CAD build for the part. Positions are in the model's coordinates, mm. Face numbers are marked on the shaded views. A direction names the side the tool comes from. Give positions to 0.01 mm unless a question says otherwise; leave off trailing zeros. Loops run counter-clockwise (first coordinate to the right, second up) from the corner with the lowest first, then second, coordinate; pieces in that order, holes last.
Item 1: Saw through at A-A on z = 14.75. Give the cut face in (x, y) (3 decimals).
Item 2: Probe probe 1 along Z at (x, y) = (-235.5, -138.5); probe 2 along X at (y, z) = (15.5, 15); probe 3 along Z at (x, y) = (-219, -82.5). List the from-to ranges inside material, lowest first.
Item 3: Drop flat-ended pins along their axis: P1, Ø3, axis at x = -22.66, y = 14.67, coming from the +Z side; P2, Ø10, axis at x = -16.5, z = 10.5, coming from the +Y side; P3, Ø10, axis at y = -122.5, z = 9, coming from the +X side; P4, Ø1.9, axis at x = -22, y = 14, coming from the +Z side. Give the stop position or say it passes through.
Item 4: Which spindle directions (+Z, -Z, +X, -X, +Y, -Y) get a long thin tool onto all of the face, cutting with end or side? Do the marked faces 1, 2 and 3. Say none if no direction does.
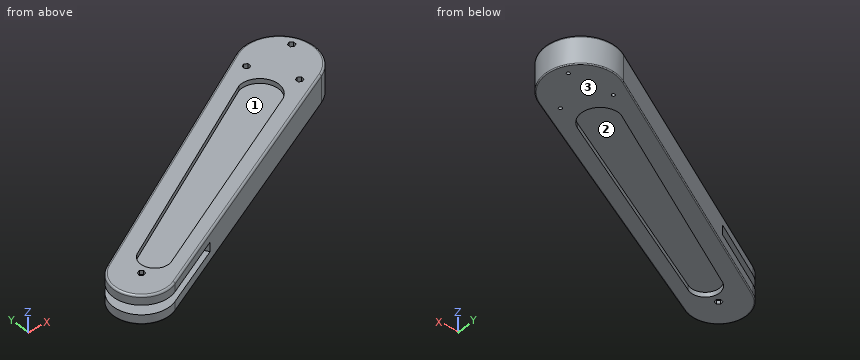
from build123d import *

# Parameters (mm, degrees)
BOSS_EXTRUDE1_DEPTH = 30
FILLET1_R           = 2
FILLET2_R           = 1
SKETCH6_W           = 100
SKETCH6_H           = 10
CUT_EXTRUDE3_DEPTH  = 129
CUT_EXTRUDE4_DEPTH  = 4
SKETCH8_R           = 1.9
CUT_EXTRUDE6_DEPTH  = 112
CUT_EXTRUDE7_DEPTH  = 5
CUT_EXTRUDE8_DEPTH  = 20
CUT_EXTRUDE9_START  = -70
SKETCH10_R          = 1.75
CUT_EXTRUDE9_DEPTH  = 71
CIRPATTERN1_COUNT   = 3


with BuildPart() as part:
    # Sketch1 → Boss-Extrude1 (new body)
    with BuildSketch(Plane.XY):
        with BuildLine():
            Line((-281.432373232, -110.20807274), (-17.900575614, 32.951773741))
            ThreePointArc((-17.900575614, 32.951773741), (33.388989093, 17.071186467), (16.23112616, -33.805333064))
            Line((16.23112616, -33.805333064), (-254.127011813, -163.613758184))
            ThreePointArc((-254.127011813, -163.613758184), (-293.823104015, -150.226440906), (-281.432373232, -110.20807274))
        make_face()
    extrude(amount=BOSS_EXTRUDE1_DEPTH)

    # Fillet1
    fillet1_edges = [part.edges().sort_by_distance(p)[0] for p in [
        (33.388989093, 17.071186467, 30),
        (-149.666474423, -38.628149499, 30),
        (-293.823104015, -150.226440906, 30),
        (-118.947942827, -98.709545624, 30),
    ]]
    fillet(fillet1_edges, radius=FILLET1_R)

    # Fillet2
    fillet2_edges = [part.edges().sort_by_distance(p)[0] for p in [
        (-149.666474423, -38.628149499, 0),
        (33.388989093, 17.071186467, 0),
        (-118.947942827, -98.709545624, 0),
        (-293.823104015, -150.226440906, 0),
    ]]
    fillet(fillet2_edges, radius=FILLET2_R)

    # Sketch6 → Cut-Extrude3 (cut)
    with BuildSketch(Plane(origin=(-17.900575614, 32.951773741, 0), x_dir=(0.8787139664263899, 0.4773486830475195, 0), z_dir=(-0.47734868304751954, 0.87871396642639, 0))):
        with Locations((-279.906235347, -15)):
            Rectangle(SKETCH6_W, SKETCH6_H)
    extrude(amount=-CUT_EXTRUDE3_DEPTH, mode=Mode.SUBTRACT)

    # Sketch7 → Cut-Extrude4 (cut)
    with BuildSketch(Plane.XY.offset(30)):
        Polygon((-263.720924854, -135.421623642), (-266.410501723, -133.058876034), (-269.80148961, -134.206744124), (-270.502900627, -137.717359822), (-267.813323758, -140.080107431), (-264.422335871, -138.932239341), align=None)
    cut_extrude4 = extrude(amount=-CUT_EXTRUDE4_DEPTH, mode=Mode.SUBTRACT)

    # Sketch8 → Cut-Extrude6 (cut)
    with BuildSketch(Plane.XY.offset(26)):
        with Locations((-267.111912741, -136.569491732)):
            Circle(SKETCH8_R)
    extrude(amount=-CUT_EXTRUDE6_DEPTH, mode=Mode.SUBTRACT)

    # Mirror1: Cut-Extrude4 across plane
    add(cut_extrude4.mirror(Plane.XY.offset(15)), mode=Mode.SUBTRACT)

    # Sketch9 → Cut-Extrude7 (cut)
    with BuildSketch(Plane.XY.offset(30)):
        with BuildLine():
            Line((-253.373411521, -115.147546234), (-44.145606003, -0.832397564))
            ThreePointArc((-44.145606003, -0.832397564), (-19.838333174, -12.433391688), (-29.122969005, -37.716233984))
            Line((-29.122969005, -37.716233984), (-237.324421153, -140.479268617))
            ThreePointArc((-237.324421153, -140.479268617), (-257.658147226, -135.611958389), (-253.373411521, -115.147546234))
        make_face()
    cut_extrude7 = extrude(amount=-CUT_EXTRUDE7_DEPTH, mode=Mode.SUBTRACT)

    # Mirror2: Cut-Extrude7 across plane
    add(cut_extrude7.mirror(Plane.XY.offset(15)), mode=Mode.SUBTRACT)

    # Sketch3 → Cut-Extrude8 (cut)
    with BuildSketch(Plane.XY.offset(30)):
        Polygon((-4.424109202, -25.18892785), (-4.53581637, -28.767184619), (-1.492808691, -30.65305425), (1.661906157, -28.96066711), (1.773613325, -25.382410341), (-1.269394354, -23.496540711), align=None)
        Polygon((27.292728029, 14.033716876), (24.249720349, 15.919586506), (21.095005502, 14.227199366), (20.983298334, 10.648942597), (24.026306013, 8.763072967), (27.181020861, 10.455460106), align=None)
        Polygon((-19.602196811, 16.425854883), (-22.645204491, 18.311724513), (-25.799919338, 16.619337374), (-25.911626506, 13.041080604), (-22.868618827, 11.155210974), (-19.713903979, 12.847598114), align=None)
    extrude(amount=-CUT_EXTRUDE8_DEPTH, mode=Mode.SUBTRACT)

    # Sketch10 → Cut-Extrude9 (cut)
    with BuildSketch(Plane.XY.offset(10).offset(CUT_EXTRUDE9_START)):
        with Locations((24.040072147, 12.291254256)):
            Circle(SKETCH10_R)
    cut_extrude9 = extrude(amount=CUT_EXTRUDE9_DEPTH, mode=Mode.SUBTRACT)

    # CirPattern1: Cut-Extrude9 ×3 about axis
    cirpattern1_axis = Axis((0, 0, 0), (0, 0, 1))
    for i in range(1, CIRPATTERN1_COUNT):
        add(cut_extrude9.rotate(cirpattern1_axis, i * 360 / CIRPATTERN1_COUNT), mode=Mode.SUBTRACT)


solid = part.part
Results below:
1. outline: (-219.922, -76.794) - (-189.591, -132.628) - (16.231, -33.805) arc R37.5 ccw (long way) to (-17.901, 32.952) - close; hole (-25.912, 13.041) - (-22.869, 11.155) - (-19.714, 12.848) - (-19.602, 16.426) - (-22.645, 18.312) - (-25.8, 16.619) - close; hole (-4.536, -28.767) - (-1.493, -30.653) - (1.662, -28.961) - (1.774, -25.382) - (-1.269, -23.497) - (-4.424, -25.189) - close; hole (20.983, 10.649) - (24.026, 8.763) - (27.181, 10.455) - (27.293, 14.034) - (24.25, 15.92) - (21.095, 14.227) - close
2. probe 1: z = 5 to 10, 20 to 25
2. probe 2: x = -50.03 to -25.83, -19.63 to 23.47, 24.93 to 34.15
2. probe 3: z = 0 to 10, 20 to 30
3. P1: passes through
3. P2: stops at y = 35.69
3. P3: stops at x = -158.08
3. P4: stops at z = 10
4. face 1: +Z
4. face 2: -Z
4. face 3: -Z, +X, -X, +Y, -Y
